Could you check a few things on this model? Use its own coordinates, in mm. A direction names the side the tool comes from. Round coordinates to 2 decimals unless told otherwise and drop trailing zeros. Order: outer loops, then holes, each group sorted by start corner. A loop starts at its lowest first (then second) coordinate and runs counter-clockwise, first axis right, second up. Notation, with made-up numbers: (-37.75, 85) -> (18.25, 85) arc R29 ccw to (18.25, 114) -> close; hole circle Ø1 at (-29, 38.25). An arc over 180 degrees is marked (long way). Put each result on its own line as item: value. Start each with the question number.
Autodesk Inventor part; units mm, degrees
ref_plane "YZ Plane" through (0, 0, 0) normal (1, 0, 0) x (0, 1, 0)
ref_plane "XZ Plane" through (0, 0, 0) normal (0, 1, 0) x (-1, 0, 0)
ref_plane "XY Plane" through (0, 0, 0) normal (0, 0, 1) x (1, 0, 0)
sketch "Sketch1" plane through (0, 0, 0) normal (0, 1, 0) x (-1, 0, 0)
  line L0 (0, 0) -> (-50, 0)
  line L1 (-50, 0) -> (-50, -120)
  line L2 (-50, -120) -> (0, -120)
  line L3 (0, -120) -> (0, 0)
  dimension "d0" = 50
  dimension "d1" = 120
extrude "Extrusion1" add sketch "Sketch1" along normal blind 10
sketch "Sketch2" plane through (0, 10, 0) normal (0, 1, 0) x (1, 0, 0)
  line L0 (0, 0) -> (50, 0)
  line L1 (50, 0) -> (50, 20)
  line L2 (50, 20) -> (0, 20)
  line L3 (0, 20) -> (0, 0)
  dimension "d4" = 50
  dimension "d5" = 20
extrude "Extrusion2" add sketch "Sketch2" along normal blind 85
chamfer "Chamfer1" distance 10 angle 45 1 edges at (25, 10, -120)
sketch "Sketch3" plane through (0, 10, 0) normal (0, 1, 0) x (1, 0, 0)
  line L0 (0, 110) -> (0, 20)
  line L1 (0, 20) -> (50, 20)
  line L2 (0, 110) -> (20, 110)
  line L3 (20, 110) -> (20, 20)
  line L4 (20, 20) -> (0, 20)
  line L5 (0, 20) -> (0, 110)
  point P0 (0, 0)
  dimension "d11" = 20
extrude "Extrusion3" add sketch "Sketch3" along normal blind 40
chamfer "Chamfer2" distance 40 angle 45 1 edges at (10, 50, -110)
fillet "Fillet1" radius 15 1 edges at (20, 30, -20)
sketch "Sketch4" plane through (50, 95, -20) normal (0, 0, -1) x (-1, 0, 0)
  point P0 (50, -95)
  point P1 (25, -20)
hole "Hole1" at (25, 75, -20) direction (0, 0, 1) diameter 20 depth 20 tip angle 118 counterbore diameter 30 counterbore depth 10
fillet "Fillet2" radius 25 2 edges at (50, 95, -10) (0, 95, -10)
sketch "Sketch5" plane through (0, 10, 0) normal (0, 1, 0) x (1, 0, 0)
  line L0 (35, 35) -> (35, 95)
  point P0 (0, 0)
  dimension "d26" = 60
hole "Hole2" at (35, 10, -35) at (35, 10, -95) direction (0, -1, 0) diameter 10 depth 10 tip angle 118 countersink diameter 20 countersink angle 90
sketch "Sketch6" plane through (50, 10, -20) normal (0, 0, -1) x (-1, 0, 0)
  line L0 (20, 79) -> (30, 79)
  line L1 (30, 79) -> (30, 86.8566)
  line L2 (30, 86.8566) -> (20, 86.8566)
  line L3 (20, 86.8566) -> (20, 79)
  point P0 (50, -10)
extrude "Extrusion4" cut sketch "Sketch6" against normal blind 10
sketch "Sketch7" plane through (20, 10, -35) normal (1, 0, 0) x (0, 0, -1)
  line L0 (5, 25) -> (40, 25)
  line L1 (40, 25) -> (40, 10)
  line L2 (40, 10) -> (5, 10)
  line L3 (5, 10) -> (5, 25)
  point P0 (-35, -10)
extrude "Extrusion5" cut sketch "Sketch7" against normal blind 20
properties part number "Part1 Drawing"
1. If we section it at C-C, the plane y = 75: Please give me the cut outline in (x, z).
2. Which directions (+Z, -Z, +X, -X, +Y, -Y) give clear straight access to the entire face, cutting with the end or side of a thin tool? Please do faces 1 (the face through (20, 92, -15)), 2 (the face through (20, 16, -65)), 3 (the face through (10, 20, -58)).
3. Thinking about a two-plate mould opening in Z: for faces 4 (the face through (35, 2, -40)), 5 (the face through (25, 47, 0)), 6 (the face through (10, 30, -90)), which applies, +Z half, -Z half, draft (parallel to the pull), parting line (faces both ways), or undercut?
4. For pin 1 Ø9 at (x, z) = (40, -61) entering from +Y; pin 2 Ø7.5 at (x, y) = (13, 29.5) entering from -Z; pin 3 Ø5 at (x, y) = (5, 59) entering from -Z, each with a flat end and sliding along its axis, tell me the tip position at first contact or that it passes through.
5. If we section it at D-D, the plane y = 16.5: Please give me the cut outline in (x, z).
6. If we section it at B-B, the plane x = 18: Count the separate pieces of the cut face and the enclosed holes in it, then the cut area to 3 significant figures.
7. I need wall thicknesses on L1, parallel to X at y = 1, z = -95; L2, parallel to Z at x = 35, y = 3.65; L3, parallel to Y at x = 15, z = -41. Which ranges of each line are inside material? Lowest first, please.
8. If we section it at A-A, the plane z = -95: Please give me the cut outline in (x, y).
Results below:
1. outline: (0.51, -20) -> (10, -20) -> (10, -10) -> (15, -10) -> (15, 0) -> (0.51, 0) -> close; (35, -10) -> (40, -10) -> (40, -20) -> (49.49, -20) -> (49.49, 0) -> (35, 0) -> close
2. face 1: -Z, +Y
2. face 2: -Z, +X, +Y
2. face 3: +X, -X
3. face 4: undercut
3. face 5: +Z half
3. face 6: -Z half
4. pin 1: y = 10
4. pin 2: z = -94.25
4. pin 3: z = -20
5. outline: (0, -103.5) -> (20, -103.5) -> (20, -35) arc R15 cw to (35, -20) -> (50, -20) -> (50, 0) -> (0, 0) -> close
6. separate pieces: 2
6. enclosed holes: 1
6. area: 4,700 mm2
7. L1: 0 to 30, 40 to 50
7. L2: -116.35 to -100, -90 to -40, -30 to 0
7. L3: 0 to 20, 35 to 50
8. outline: (0, 0) -> (30, 0) -> (30, 5) -> (25, 10) -> (20, 10) -> (20, 25) -> (0, 25) -> close; (40, 0) -> (50, 0) -> (50, 10) -> (45, 10) -> (40, 5) -> close
